```python
from build123d import *

# Parameters (mm, degrees)
SKETCH_R     = 1.8
PAD_DEPTH    = 1
CHAMFER_SIZE = 0.99


with BuildPart() as part:
    # Sketch → Pad (new body)
    with BuildSketch(Plane.XZ):
        with BuildLine():
            Line((6.75, 38), (6.75, 0))
            ThreePointArc((-6.75, 0), (0, -6.75), (6.75, 0))
            Line((-6.75, 0), (-6.75, 38))
            ThreePointArc((6.75, 38), (0, 44.75), (-6.75, 38))
        make_face()
        with Locations((0, 38)):
            Circle(SKETCH_R, mode=Mode.SUBTRACT)
        Circle(SKETCH_R, mode=Mode.SUBTRACT)
    extrude(amount=PAD_DEPTH)

    # Chamfer
    chamfer_edges = [part.edges().sort_by_distance(p)[0] for p in [
        (-1.8, 0, 0),
        (-1.8, 0, 38),
    ]]
    chamfer(chamfer_edges, length=CHAMFER_SIZE)


solid = part.part
```
Input: part model. Units: mm. Frame: model coordinates. Coordinates: 2 decimals unless noted, no trailing zeros. Write each loop counter-clockwise with the first axis right and the second up, starting at its lowest first coordinate (ties: lowest second). Pieces come first, ordered by that corner, then holes. Notation, with made-up numbers: (-18.75, -8) -> (35.25, -8) arc R22 cw to (35.25, 21) -> close; hole circle Ø8 at (86, -22). An arc over 180 degrees is marked (long way). Answer as a JSON object with one key per item and string values.
1. Section B-B on x = 0. Count the separate pieces of the cut face and the enclosed holes in it, then the cut area to 3 significant figures.
Result set:
{"separate pieces": "3", "enclosed holes": "0", "area": "42.3 mm2"}
2. Section C-C on x = -4.5. Return the cut outline in (y, z).
Result set:
{"outline": "(-1, -5.03) -> (0, -5.03) -> (0, 43.03) -> (-1, 43.03) -> close"}
3. Material intervals for line 1 (Z direction, x = 0.5, y = -0.9); line 2 (X direction, y = -0.35, z = 1); line 3 (X direction, y = -0.05, z = 36), sorted ascending. Write a range as from..to.
Result set:
{"line 1": "z = -6.73..-1.82, 1.82..36.18, 39.82..44.73", "line 2": "x = -6.75..-2.23, 2.23..6.75", "line 3": "x = -6.75..-1.87, 1.87..6.75"}
4. Section A-A on y = -0.7. Return the cut outline in (x, z).
Result set:
{"outline": "(-6.75, 0) arc R6.75 ccw to (6.75, 0) -> (6.75, 38) arc R6.75 ccw to (-6.75, 38) -> close; hole circle Ø4.18 at (0, 0); hole circle Ø4.18 at (0, 38)"}
